For this review, take the finished solid that the model builds, in its own axes (mm). A direction names the side the tool comes from. Coordinates: 2 decimals unless noted, no trailing zeros. Order: outer loops, then holes, each group sorted by start corner. A loop starts at its lowest first (then second) coordinate and runs counter-clockwise, first axis right, second up. Notation, with made-up numbers: (25.25, 67) -> (57.25, 67) arc R21 cw to (57.25, 76) -> close; hole circle Ø6 at (-27, -36.5). An arc over 180 degrees is marked (long way). Return JSON: item names as keys, results as strings. Group by question number.
Item 1: Take a section at A-A (x = -47). Write out the cut boundary in (y, z).
Item 2: Draft analysis for pull direction Y (two halves, no side actions). For faces 1 (the flat face through (49, 0, 0)), 2 (the cylindrical face through (155.69, 52.19, 2.82)), 3 (the flat face through (-15, 72, 6)), state which applies: +Y half, -Y half, draft (parallel to the pull), parting line (faces both ways), or undercut.
Item 3: Machinability: for faces 4 (the conical face through (150.99, 101.13, 10.42)), 5 (the flat face through (159, 103, 0)), 6 (the flat face through (-6, 137, -6)), 7 (the cylindrical face through (60.553, 122.892, 6.042)), which of the approach directions +Z, -Z, +X, -X, +Y, -Y give a long, thin tool a straight path to every point of the face, cutting with its end or side? Answer none if there is none.
Item 4: Take a section at C-C (z = 0). Write out the cut boundary in (x, y).
Item 5: For line 1 along X through (y, z) = (53.5, 0); line 2 along X through (y, z) = (89, -10.5); line 3 along Z through (x, y) = (143, 63), list the stretches that pass through material, from the lowest coordinate up.
Item 6: Take a section at D-D (y = 90.5). Write out the cut boundary in (x, z).
Item 7: Take a section at B-B (y = 48). Write out the cut boundary in (x, z).
Item 8: Insertion check: pin 1 (3 mm diameter, centred on x = 20.5, z = 6.5, fed in from +Y); pin 2 (3 mm diameter, centred on x = -24.5, z = 15.5, fed in from +Y); pin 3 (5 mm diameter, centred on y = 105.5, z = -3, fed in from -X) (3 decimals); pin 4 (1.8 mm diameter, centred on y = 32, z = 6.5, fed in from -X). Each pin has a flat end and moves straight along its axis. Give the tip position at first contact, or say it passes through.
```python
from build123d import *

# Parameters (mm, degrees)
SKETCH1_W                = 18
SKETCH1_H                = 103
SKETCH3_W                = 12
SKETCH3_H                = 143
CHAMFER1_SIZE            = 2
CHAMFER2_SIZE            = 2
FILLET1_R                = 2
FILLET2_R                = 2
FILLET3_R                = 7
BOSS_EXTRUDE1_DEPTH      = 9
BOSS_EXTRUDE1_DEPTH_BACK = 9
CUT_EXTRUDE1_DEPTH       = 6


with BuildPart() as part:
    # Sketch1 → Revolve2 (revolve)
    with BuildSketch(Plane.XY, mode=Mode.PRIVATE) as revolve2_sk:
        with Locations((165, 51.5)):
            Rectangle(SKETCH1_W, SKETCH1_H)
    revolve(revolve2_sk.sketch.rotate(Axis((143, 0, 0), (0, 1, 0)), 90), axis=Axis((143, 0, 0), (0, 1, 0)))

    # Chamfer2
    chamfer2_edges = [part.edges().sort_by_distance(p)[0] for p in [
        (143, 103, 13),
        (143, 0, 13),
    ]]
    chamfer(chamfer2_edges, length=CHAMFER2_SIZE)

    # Fillet2
    fillet2_edges = [part.edges().sort_by_distance(p)[0] for p in [
        (143, 0, 31),
    ]]
    fillet(fillet2_edges, radius=FILLET2_R)

    # Fillet3
    fillet3_edges = [part.edges().sort_by_distance(p)[0] for p in [
        (143, 103, 31),
    ]]
    fillet(fillet3_edges, radius=FILLET3_R)



with BuildPart() as body_2:
    # Sketch3 → Revolve3 (revolve)
    with BuildSketch(Plane.XY, mode=Mode.PRIVATE) as revolve3_sk:
        with Locations((-66, 71.5)):
            Rectangle(SKETCH3_W, SKETCH3_H)
    revolve(revolve3_sk.sketch.rotate(Axis((-47, 0, 0), (0, 1, 0)), 270), axis=Axis((-47, 0, 0), (0, 1, 0)))

    # Chamfer1
    chamfer1_edges = [body_2.edges().sort_by_distance(p)[0] for p in [
        (-47, 143, 13),
        (-47, 0, 13),
    ]]
    chamfer(chamfer1_edges, length=CHAMFER1_SIZE)

    # Fillet1
    fillet1_edges = [body_2.edges().sort_by_distance(p)[0] for p in [
        (-47, 143, 25),
        (-47, 0, 25),
    ]]
    fillet(fillet1_edges, radius=FILLET1_R)


with BuildPart() as part_1:
    add(part.part)

    add(body_2.part)  # Boss-Extrude1 merges body 2
    # Sketch4 → Boss-Extrude1 (add, two sides: drawn at the far end of the back side and taken through both)
    with BuildSketch(Plane.XY.offset(-BOSS_EXTRUDE1_DEPTH_BACK)):
        with BuildLine():
            Line((0, 0), (-27.193276933, 0))
            Line((-27.193276933, 0), (-27.193276933, 143))
            Line((-27.193276933, 143), (0, 143))
            ThreePointArc((0, 143), (69.368060127, 125.048279613), (121.319672434, 75.700310967))
            Line((121.319672434, 75.700310967), (121.319672434, 0))
            Line((121.319672434, 0), (0, 0))
        make_face()
    extrude(amount=BOSS_EXTRUDE1_DEPTH + BOSS_EXTRUDE1_DEPTH_BACK)

    # Sketch6 → Cut-Extrude1 (cut)
    with BuildSketch(Plane.XY.offset(9)):
        with BuildLine():
            Line((0, 137), (-13, 137))
            ThreePointArc((-13, 137), (-14.414213562, 136.414213562), (-15, 135))
            Line((-15, 135), (-15, 8))
            ThreePointArc((-15, 8), (-14.414213562, 6.585786438), (-13, 6))
            Line((-13, 6), (106, 6))
            ThreePointArc((106, 6), (107.414213562, 6.585786438), (108, 8))
            Line((108, 8), (108, 83.600239234))
            ThreePointArc((108, 83.600239234), (107.889542371, 84.255700621), (107.57037037, 84.838761297))
            ThreePointArc((107.57037037, 84.838761297), (59.774951704, 123.27187493), (0, 137))
        make_face()
    cut_extrude1 = extrude(amount=-CUT_EXTRUDE1_DEPTH, mode=Mode.SUBTRACT)

    # Mirror1: Cut-Extrude1 across plane
    add(cut_extrude1.mirror(Plane.XY), mode=Mode.SUBTRACT)


solid = part_1.part
```
Findings below:
{
 "1": {"outline": "(0, -23) arc R2 ccw to (2, -25) -> (141, -25) arc R2 ccw to (143, -23) -> (143, -15) -> (141, -13) -> (2, -13) -> (0, -15) -> close; (0, 15) -> (2, 13) -> (141, 13) -> (143, 15) -> (143, 23) arc R2 ccw to (141, 25) -> (2, 25) arc R2 ccw to (0, 23) -> close"},
 "2": {"face 1": "-Y half", "face 2": "draft", "face 3": "undercut"},
 "3": {"face 4": "+Y", "face 5": "+Z, -Z, +X, +Y", "face 6": "-Z", "face 7": "+Z"},
 "4": {"outline": "(-72, 2) arc R2 ccw to (-70, 0) -> (-62, 0) -> (-60, 2) -> (-60, 141) -> (-62, 143) -> (-70, 143) arc R2 ccw to (-72, 141) -> close; (-34, 2) -> (-32, 0) -> (128, 0) -> (130, 2) -> (130, 101) -> (128, 103) -> (119, 103) arc R7 ccw to (112, 96) -> (112, 88.91) arc R143 ccw to (0, 143) -> (-32, 143) -> (-34, 141) -> close; (156, 2) -> (158, 0) -> (172, 0) arc R2 ccw to (174, 2) -> (174, 96) arc R7 ccw to (167, 103) -> (158, 103) -> (156, 101) -> close"},
 "5": {"line 1": "x = -72 to -60, -34 to 130, 156 to 174", "line 2": "x = -69.69 to -54.66, -39.34 to -24.31, 113.83 to 135.34, 150.66 to 172.17", "line 3": "z = -31 to -13, 13 to 31"},
 "6": {"outline": "(-23.68, -9) -> (-15, -9) -> (-15, -3) -> (102.85, -3) -> (102.85, -9) -> (110.72, -9) -> (110.72, 9) -> (102.85, 9) -> (102.85, 3) -> (-15, 3) -> (-15, 9) -> (-23.68, 9) arc R25 ccw (long way) to start; circle Ø62 at (143, 0); hole circle Ø26 at (-47, 0); hole circle Ø26 at (143, 0)"},
 "7": {"outline": "(-23.68, -9) -> (-15, -9) -> (-15, -3) -> (108, -3) -> (108, -9) -> (113.34, -9) arc R31 ccw (long way) to (113.34, 9) -> (108, 9) -> (108, 3) -> (-15, 3) -> (-15, 9) -> (-23.68, 9) arc R25 ccw (long way) to start; hole circle Ø26 at (-47, 0); hole circle Ø26 at (143, 0)"},
 "8": {"pin 1": "stops at y = 141.73", "pin 2": "passes through", "pin 3": "stops at x = -71.995", "pin 4": "stops at x = -71.36"}
}
